from build123d import *

# Parameters (mm, degrees)
SKETCH_6_W             = 51
SKETCH_6_H             = 38
EXTRUDE_647_DEPTH      = 11
SKETCH_10_R            = 10
EXTRUDE_856_DEPTH      = 3
FILLET_1_R             = 3
SKETCH_13_R            = 1.25
CUT_EXTRUDE_1173_DEPTH = 52
SKETCH_15_R            = 8.65
EXTRUDE_1309_DEPTH     = 13
CUT_EXTRUDE_START      = -13
CUT_EXTRUDE_1600_DEPTH = 13
SKETCH_26_R            = 1.65
CUT_EXTRUDE_1838_DEPTH = 39.961519478
CHAMFER_7_SIZE         = 2
SKETCH_17_R            = 3
CUT_EXTRUDE_2253_DEPTH = 46.287967497
SKETCH_19_W            = 14
SKETCH_19_H            = 38
EXTRUDE_2866_DEPTH     = 2
SKETCH_20_R            = 1.65
CUT_EXTRUDE_3095_DEPTH = 44.886216515
SKETCH_23_R            = 5
SKETCH_23_R_2          = 1.65
EXTRUDE_3300_DEPTH     = 2
CHAMFER_4_SIZE         = 1
FILLET_7_R             = 3
CHAMFER_6_SIZE         = 1.5
FILLET_8_R             = 0.5


with BuildPart() as part:
    # Эскиз6 → Extrude 647 (new body)
    with BuildSketch(Plane(origin=(0, 0, 0), x_dir=(1, 0, 0), z_dir=(0, 1, 0))):
        with Locations((5.5, 0)):
            Rectangle(SKETCH_6_W, SKETCH_6_H)
    extrude(amount=EXTRUDE_647_DEPTH)

    # Эскиз10 → Extrude 856 (add)
    with BuildSketch(Plane(origin=(0, 11, 0), x_dir=(1, 0, 0), z_dir=(0, 1, 0))):
        with Locations(Location((0, 0, 0), (0, 0, 90))):
            Circle(SKETCH_10_R)
    extrude(amount=EXTRUDE_856_DEPTH)

    # Скругление1
    fillet_1_edges = [part.edges().sort_by_distance(p)[0] for p in [
        (0, 11, 10),
    ]]
    fillet(fillet_1_edges, radius=FILLET_1_R - 0.0001)  # a hair under: the kernel refuses the full size

    # Эскиз13 → Cut-Extrude 1173 (cut, through all)
    with BuildSketch(Plane.XY.offset(19)):
        with Locations((-13, 5.5)):
            Circle(SKETCH_13_R)
        with Locations((13, 5.5)):
            Circle(SKETCH_13_R)
    extrude(amount=-CUT_EXTRUDE_1173_DEPTH, mode=Mode.SUBTRACT)

    # Эскиз15 → Extrude 1309 (add)
    with BuildSketch(Plane(origin=(0, 14, 0), x_dir=(1, 0, 0), z_dir=(0, 1, 0))):
        with Locations(Location((0, 0, 0), (0, 0, 90))):
            Circle(SKETCH_15_R)
    extrude(amount=EXTRUDE_1309_DEPTH)

    # Эскиз16 → Cut-Extrude 1600 (cut)
    with BuildSketch(Plane(origin=(0, 27, 0), x_dir=(1, 0, 0), z_dir=(0, 1, 0)).offset(CUT_EXTRUDE_START)):
        with BuildLine():
            Line((-1.65, 7), (-1.65, 8.491171886))
            ThreePointArc((-1.65, 8.491171886), (0, 8.65), (1.65, 8.491171886))
            Line((1.65, 8.491171886), (1.65, 7))
            ThreePointArc((1.65, 7), (0, 5.35), (-1.65, 7))
        make_face()
        with BuildLine():
            Line((1.65, -7), (1.65, -8.491171886))
            ThreePointArc((1.65, -8.491171886), (0, -8.65), (-1.65, -8.491171886))
            Line((-1.65, -8.491171886), (-1.65, -7))
            ThreePointArc((-1.65, -7), (0, -5.35), (1.65, -7))
        make_face()
    extrude(amount=CUT_EXTRUDE_1600_DEPTH, mode=Mode.SUBTRACT)

    # Эскиз26 → Cut-Extrude 1838 (cut, through all)
    with BuildSketch(Plane(origin=(0, 14, 0), x_dir=(1, 0, 0), z_dir=(0, 1, 0))):
        with Locations(Location((0, 7, 0), (0, 0, 270))):
            Circle(SKETCH_26_R)
        with Locations(Location((0, -7, 0), (0, 0, 270))):
            Circle(SKETCH_26_R)
    extrude(amount=-CUT_EXTRUDE_1838_DEPTH, mode=Mode.SUBTRACT)

    # Фаска7
    chamfer_7_edges = [part.edges().sort_by_distance(p)[0] for p in [
        (0, 0, -8.65),
        (0, 0, 5.35),
    ]]
    chamfer(chamfer_7_edges, length=CHAMFER_7_SIZE)

    # Эскиз17 → Cut-Extrude 2253 (cut, through all)
    with BuildSketch(Plane(origin=(0, 27, 0), x_dir=(1, 0, 0), z_dir=(0, 1, 0))):
        with Locations(Location((0, 0, 0), (0, 0, 270))):
            Circle(SKETCH_17_R)
    extrude(amount=-CUT_EXTRUDE_2253_DEPTH, mode=Mode.SUBTRACT)

    # Эскиз19 → Extrude 2866 (add)
    with BuildSketch(Plane(origin=(0, 11, 0), x_dir=(1, 0, 0), z_dir=(0, 1, 0))):
        with Locations((30, 0)):
            Rectangle(SKETCH_19_W, SKETCH_19_H)
    extrude(amount=EXTRUDE_2866_DEPTH)

    # Эскиз20 → Cut-Extrude 3095 (cut, through all)
    with BuildSketch(Plane(origin=(0, 13, 0), x_dir=(1, 0, 0), z_dir=(0, 1, 0))):
        with Locations(Location((34, 10, 0), (0, 0, 270))):
            Circle(SKETCH_20_R)
        with Locations(Location((34, -10, 0), (0, 0, 270))):
            Circle(SKETCH_20_R)
    extrude(amount=-CUT_EXTRUDE_3095_DEPTH, mode=Mode.SUBTRACT)

    # Эскиз23 → Extrude 3300 (add)
    # profile 1 of 2: a face of its own
    with BuildSketch(Plane(origin=(0, 13, 0), x_dir=(1, 0, 0), z_dir=(0, 1, 0))):
        with Locations((34, 10)):
            Circle(SKETCH_23_R)
        with Locations(Location((34, 10, 0), (0, 0, 270))):
            Circle(SKETCH_23_R_2, mode=Mode.SUBTRACT)
    # profile 2 of 2: a face of its own
    with BuildSketch(Plane(origin=(0, 13, 0), x_dir=(1, 0, 0), z_dir=(0, 1, 0))):
        with Locations((34, -10)):
            Circle(SKETCH_23_R)
        with Locations(Location((34, -10, 0), (0, 0, 270))):
            Circle(SKETCH_23_R_2, mode=Mode.SUBTRACT)
    extrude(amount=-EXTRUDE_3300_DEPTH)

    # Фаска4
    chamfer_4_edges = [part.edges().sort_by_distance(p)[0] for p in [
        (23, 11, 0),
    ]]
    chamfer(chamfer_4_edges, length=CHAMFER_4_SIZE)
    chamfer_4_2_edges = [part.edges().sort_by_distance(p)[0] for p in [
        (23, 13, 0),
    ]]
    chamfer(chamfer_4_2_edges, length=CHAMFER_4_SIZE - 0.0001)  # a hair under: the kernel refuses the full size

    # Скругление7
    fillet_7_edges = [part.edges().sort_by_distance(p)[0] for p in [
        (23.9999, 13, 0),
        (22, 11, 0),
    ]]
    fillet(fillet_7_edges, radius=FILLET_7_R)

    # Фаска6
    chamfer_6_edges = [part.edges().sort_by_distance(p)[0] for p in [
        (34, 13, -11.65),
        (34, 13, 8.35),
    ]]
    chamfer(chamfer_6_edges, length=CHAMFER_6_SIZE)

    # Скругление8
    fillet_8_edges = [part.edges().sort_by_distance(p)[0] for p in [
        (-1.65, 20.5, -8.491171886),
        (1.65, 20.5, -8.491171886),
        (1.65, 20.5, 8.491171886),
        (-1.65, 20.5, 8.491171886),
    ]]
    fillet(fillet_8_edges, radius=FILLET_8_R)


solid = part.part
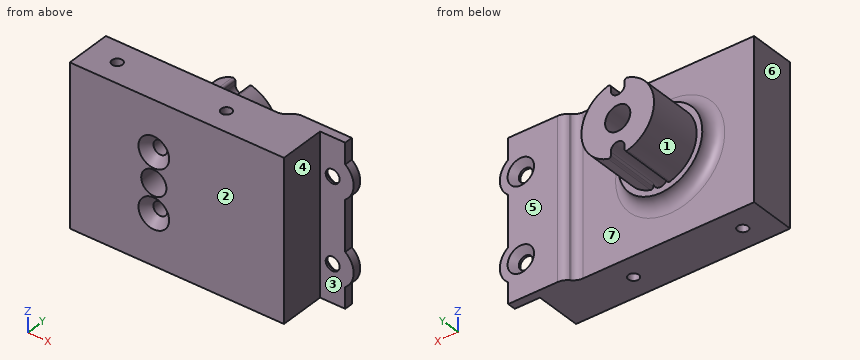
Check sheet for the modelled part. Datum: model origin and axes. Units: mm. Face numbers are marked on the shaded views. A direction names the side the tool comes from. Round coordinates to 2 decimals unless told otherwise and drop trailing zeros. Loops run counter-clockwise (first coordinate to the right, second up) from the corner with the lowest first, then second, coordinate; pieces in that order, holes last.
1. Mould release check, pull along X, two halves, no side actions. Record for the marked faces 4, 5, 6 and 7: released by +X, released by -X, zero draft, split by the parting line, or undercut.
2. Set-up check for the marked faces 1, 2 and 3: record each of +Z, -Z, +X, -X, +Y, -Y from which the full face is reachable in a straight line by a thin tool's end or side.
3. Gauge pin test, flat ends, axial feed: pin 1 Ø3 at (x, z) = (12.5, -8) entering from -Y; pin 2 Ø2 at (x, z) = (0, -7) entering from +Y; pin 3 Ø2.5 at (x, z) = (36.5, 4) entering from -Y; pin 4 Ø6 at (x, z) = (16, 1.5) entering from +Y. Record the tip position at first contact, or that the pin passes through.
4. Sectioned sample at D-D on y = 15.25. Record the boundary of the cut face in (x, z).
5. Sectioned sample at A-A on z = 0. Give the number of separate pieces and of enclosed holes in the cut face, and give its area (3 significant figures).
6. Sectioned sample at C-C on x = 34. Record the boundary of the cut face in (y, z).
7. Sectioned sample at B-B on y = 5.5. Record the boundary of the cut face in (x, z).
8. Scan lines: probe 1 along X at (y, z) = (10, 7); probe 2 along X at (y, z) = (12.25, 0); probe 3 along Y at (x, z) = (-13, -5). Record each from-to range of solid material in increasing order.
Recorded:
1. face 4: released by +X
1. face 5: zero draft
1. face 6: released by -X
1. face 7: undercut
2. face 1: -X, +Y
2. face 2: +Z, -Z, +X, -X, -Y
2. face 3: +Z, -Z, +X, -Y
3. pin 1: stops at y = 0
3. pin 2: passes through
3. pin 3: stops at y = 11
3. pin 4: stops at y = 11
4. outline: (-2.28, -8.34) arc R0.5 ccw to (-1.65, -7.86) - (-1.65, -7) arc R1.65 cw to (1.65, -7) - (1.65, -7.86) arc R0.5 ccw to (2.28, -8.34) arc R8.65 ccw to (2.28, 8.34) arc R0.5 ccw to (1.65, 7.86) - (1.65, 7) arc R1.65 cw to (-1.65, 7) - (-1.65, 7.86) arc R0.5 ccw to (-2.28, 8.34) arc R8.65 ccw to start; hole circle Ø6 at (0, 0)
5. separate pieces: 2
5. enclosed holes: 2
5. area: 706 mm2
6. outline: (11, -19) - (13, -19) - (13, -13.15) - (11.5, -11.65) - (11, -11.65) - close; (11, -8.35) - (11.5, -8.35) - (13, -6.85) - (13, 6.85) - (11.5, 8.35) - (11, 8.35) - close; (11, 11.65) - (11.5, 11.65) - (13, 13.15) - (13, 19) - (11, 19) - close
7. outline: (-20, -19) - (-14.25, -19) - (-14.25, 19) - (-20, 19) - close; (-11.75, -19) - (11.75, -19) - (11.75, 19) - (-11.75, 19) - close; (14.25, -19) - (31, -19) - (31, 19) - (14.25, 19) - close; hole circle Ø6 at (0, 0); hole circle Ø3.3 at (0, -7); hole circle Ø3.3 at (0, 7)
8. probe 1: x = -20 to -1.65, 1.65 to 31
8. probe 2: x = -10.56 to -3, 3 to 10.56, 23.26 to 37
8. probe 3: y = 0 to 4.25, 6.75 to 11
